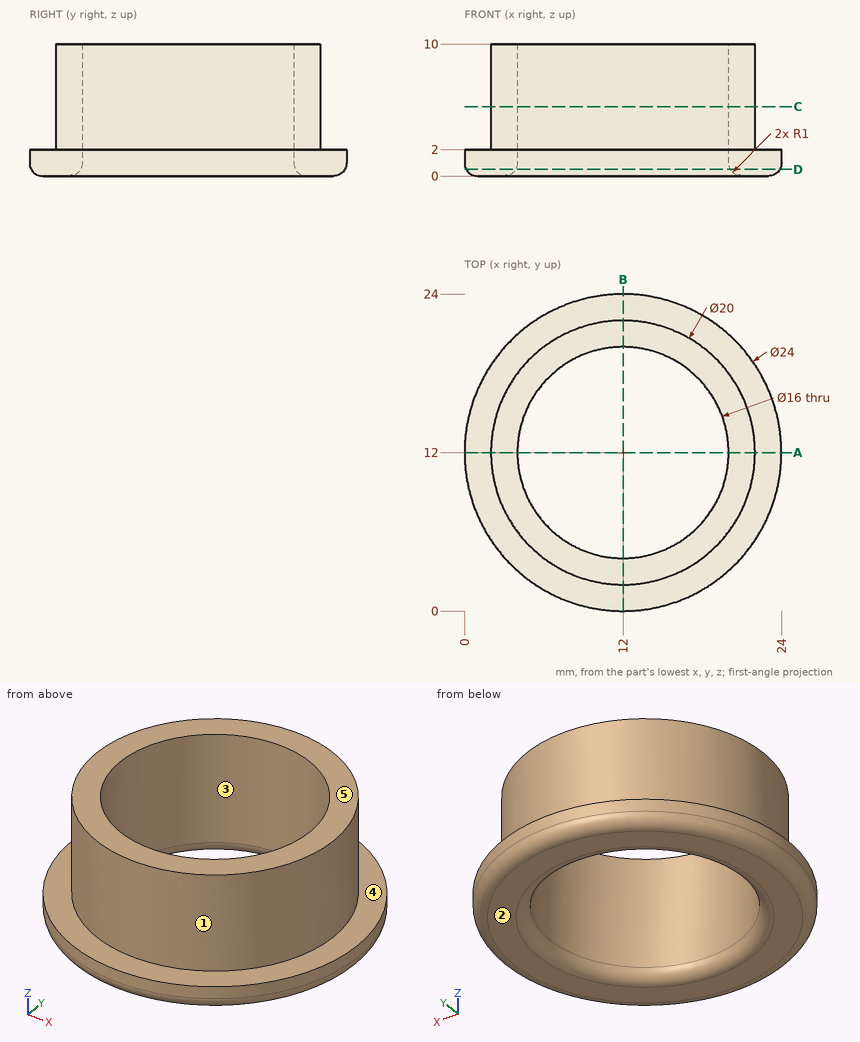
Here's the drawing with two shaded views (mm, measured from the low corner). I have some questions. A direction names the side the tool comes from. Coordinates: 2 decimals unless noted, no trailing zeros. Write each loop counter-clockwise with the first axis right and the second up, starting at its lowest first coordinate (ties: lowest second). Pieces come first, ordered by that corner, then holes. Notation, with made-up numbers: M 28.25,59.5 L 87.25,59.5 A8 ccw 87.25,65.5 Z; hole C 38.25,75 d7. An arc over 180 degrees is marked long. Answer as CSV lines item,"result". Start each with the question number.
1) We'd pull the mould along X, two halves only. Please class the marked faces 1, 2 and 3: +X half, -X half, draft (parallel to the pull), parting line (faces both ways), or undercut.
2) I want a section at A-A, the plane y = 12. Please give me the cut outline in (x, z).
3) I want a section at D-D, the plane z = 0.5. Please give me the cut outline in (x, y), and give its area (3 significant figures).
4) I want a section at C-C, the plane z = 5.25. Please give me the cut outline in (x, y), and give its area (3 significant figures).
5) For the marked faces 4 and 5, which set-ups out of +Z, -Z, +X, -X, +Y, -Y let a thin tool reach every point of the face, with its end or its side?
6) Please list where these lines run through material, in increasing order: line 1 (Y direction, x = 12, z = 5.75); line 2 (Z direction, x = 19.5, y = 19.5); line 3 (Y direction, x = 9, z = 9.75). Write a range as from..to.
7) For P1, Ø6, axis at y = 20.5, z = 5.5, coming from the +X side; P2, Ø5, axis at x = 13, z = 8.5, coming from the -Y side; P3, Ø2, axis at x = 9.5, z = 5, coming from the -Y side; P4, Ø2, axis at x = 6, y = 14, coming from the -Z side, each with a flat end and sliding along its axis, tell me the tip position at first contact or that it passes through.
Data:
1,face 1,"parting line"
1,face 2,"draft"
1,face 3,"undercut"
2,outline,"M 0,1 A1 ccw 1,0 L 3,0 A1 ccw 4,1 L 4,10 L 2,10 L 2,2 L 0,2 Z; M 20,1 A1 ccw 21,0 L 23,0 A1 ccw 24,1 L 24,2 L 22,2 L 22,10 L 20,10 Z"
3,outline,"C 12,12 d23.73; hole C 12,12 d16.27"
3,area,"234 mm^2"
4,outline,"C 12,12 d20; hole C 12,12 d16"
4,area,"113 mm^2"
5,face 4,"+Z"
5,face 5,"+Z, +X, -X, +Y, -Y"
6,line 1,"y = 2..4, 20..22"
6,line 2,"z = 0..2"
6,line 3,"y = 2.46..4.58, 19.42..21.54"
7,P1,"stops at x = 20.35"
7,P2,"stops at y = 2"
7,P3,"stops at y = 2.11"
7,P4,"passes through"
